Autodesk Inventor part; units mm, degrees
ref_plane "Work Plane6" through (-3.713488, 14.864291, 104.198762) normal (0, 0, 1) x (0.9994468, -0.0332592, 0)
ref_plane "YZ Plane" through (0, 0, 0) normal (1, 0, 0) x (0, 1, 0)
ref_plane "XZ Plane" through (0, 0, 0) normal (0, 1, 0) x (-1, 0, 0)
ref_plane "Work Plane6" through (-3.713488, 14.864291, 104.198762) normal (0, 0, 1) x (0.9994468, -0.0332592, 0)
sketch "Sketch1" plane through (-3.713488, 14.864291, 104.198762) normal (0, 0, 1) x (0.9994468, -0.0332592, 0)
  arc A0 (131.880776, 188.685572) -> (21.678185, -9.803405) centre (53.87003, 102.160585) ccw
  line L0 (131.880776, 188.685572) -> (436.873817, -86.295513)
  circle A1 centre (53.87003, 102.160585) radius 17.5
  arc A2 (21.678185, -9.803405) -> (24.529382, -10.584155) centre (53.87003, 102.160585) ccw
  arc A3 (421.49686, -114.765827) -> (436.873817, -86.295513) centre (425.724642, -98.66153) ccw
  line L1 (21.678185, -9.803405) -> (421.49686, -114.765827)
ref_plane "Work Plane13" through (20.450302, 3.470164, 104.198762) normal (0.9582447, -0.2859495, 0) x (0.2859495, 0.9582447, 0)
sketch "Sketch2" plane through (82.301795, 210.740594, 104.198762) normal (0.9582447, -0.2859495, 0) x (0.2859495, 0.9582447, 0)
  line L0 (-213.329407, -5) -> (-219.329407, -5)
  line L1 (-219.329407, -5) -> (-219.329407, 5)
  line L2 (-219.329407, 5) -> (-213.329407, 5)
  line L3 (-213.329407, 5) -> (-213.329407, -5)
  line L4 (-219.329407, -5) -> (-213.329407, 5) construction
  line L5 (-219.329407, 5) -> (-213.329407, -5) construction
  point P0 (-216.329407, 0)
  point P1 (-216.329407, 0)
  point P2 (-216.329407, 0)
  point P3 (-216.329407, 0)
  dimension "d0" = 6
  dimension "d1" = 10
sweep "Sweep1" add profiles "Sketch2" path "Sketch1" path curves L1 A3 L0 A0
properties part number "Cadena2"
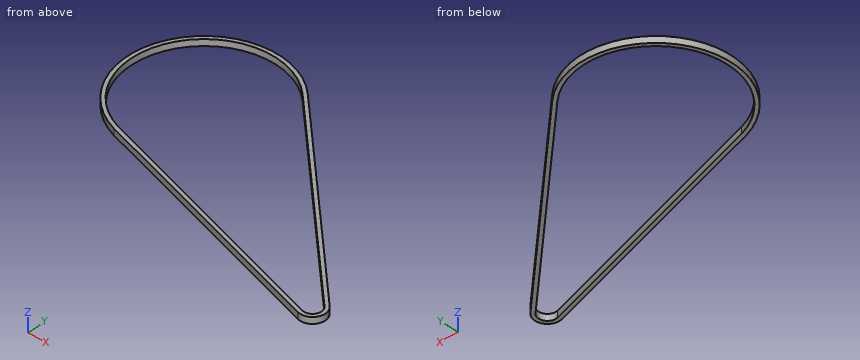
The model under review builds one solid part; all positions refer to its coordinate system, in mm. Coordinates: 2 decimals unless noted, no trailing zeros. Write each loop counter-clockwise with the first axis right and the second up, starting at its lowest first coordinate (ties: lowest second). Pieces come first, ordered by that corner, then holes. Notation, with made-up numbers: (28, 50.5) - (55, 50.5) arc R7 ccw to (55, 55.5) - close; hole circle Ø1 at (5.5, 52). An arc over 180 degrees is marked (long way). Answer in a Markdown table with one row per item. Add a question column.
Q1. Consider section B-B on x = 257. Give the boundary of the cut face in (y, z).
Q2. To check wall thickness, follow line 1 along X through (y, z) = (90.5, 106.5); line 2 along X through (y, z) = (30, 106.75); line 3 along Y through (x, z) = (362, 100). State the ranges of each line that lie inside material, in increasing order. Write a range as from..to.
Q3. Clearance check with flat-ended pins moving along their axes: pin 1 (3 mm diameter, centred on x = 327.5, z = 103, fed in from -Y); pin 2 (1.5 mm diameter, centred on y = 165, z = 105, fed in from -X); pin 3 (1 mm diameter, centred on x = 282.5, z = 104, fed in from +Y). State where each tip first meets the part, or that it passes through.
Q4. Consider section A-A on y = 157. Give the boundary of the cut face in (x, z).
Answers below:
| question | item | result |
|---|---|---|
| 1 | outline | (-70.28, 99.2) - (-64.02, 99.2) - (-64.02, 109.2) - (-70.28, 109.2) - close; (76.78, 99.2) - (85.12, 99.2) - (85.12, 109.2) - (76.78, 109.2) - close |
| 2 | line 1 | -63.46..-57.32, 242.77..251.41 |
| 2 | line 2 | -30.38..-21.58, 305.54..314.19 |
| 2 | line 3 | -101.61..-95.35, -24.41..-16.08 |
| 3 | pin 1 | y = -91.76 |
| 3 | pin 2 | x = -55.5 |
| 3 | pin 3 | y = 61.02 |
| 4 | outline | (-58.48, 99.2) - (-52.05, 99.2) - (-52.05, 109.2) - (-58.48, 109.2) - close; (173.77, 99.2) - (182.42, 99.2) - (182.42, 109.2) - (173.77, 109.2) - close |
